from build123d import *

# Parameters (mm, degrees)
REVOLVE1_ANGLE = 180
SHELL1_START   = -239.158306138
SHELL1_DEPTH   = 42.206593174
SHELL1_START_2 = -3.058115052
SHELL1_2_DEPTH = 41.216014124
SHELL1_START_3 = -196.951712964
SHELL1_3_DEPTH = 193.893597912
SHELL1_START_4 = -221.288155922
SHELL1_4_DEPTH = 5.892364499


# Read off the part's stored shape, not the designer's step: Shell1
with BuildPart() as part:
    # Sketch1 → Revolve1 (revolve)
    with BuildSketch(Plane.XY):
        Polygon((89.874416534, -245.158306138), (12.7, -245.158306138), (12.7, -242.138884915), (26.163339875, -242.138884915), (26.163339875, -227.288155922), (13.03850974, -227.288155922), (13.03850974, -209.395791423), (26.163339875, -209.395791423), (26.163339875, -194.322320246), (13.03850974, -194.322320246), (13.03850974, -190.951712964), (73.402730944, -190.951712964), (73.402730944, -136.120329582), (15.924443856, -136.120329582), (15.924443856, -125.873058549), (73.402730944, -125.873058549), (73.402730944, -72.501855253), (16.640249143, -72.501855253), (16.640249143, -62.681553847), (73.402730944, -62.681553847), (73.402730944, -9.058115052), (18.31208302, -9.058115052), (18.31208302, -7.976977068), (29.551500324, -7.976977068), (29.551500324, 8.480345585), (18.31208302, 8.480345585), (18.31208302, 18.090461002), (29.551500324, 18.090461002), (29.551500324, 35.26854231), (18.31208302, 35.26854231), (18.31208302, 44.157899072), (89.874416534, 44.157899072), align=None)
    revolve(axis=Axis((0, 19.84375, 0), (0, 1, 0)), revolution_arc=REVOLVE1_ANGLE)

    # Shell1 outline → Shell1 (cut)
    with BuildSketch(Plane(origin=(0, 0, 0), x_dir=(1, 0, 0), z_dir=(0, 1, 0)).offset(SHELL1_START)):
        with BuildLine():
            ThreePointArc((83.874416534, 0), (0, 83.874416534), (-83.874416534, 0))
            Line((-83.874416534, 0), (-32.163339875, 0))
            ThreePointArc((-32.163339875, 0), (0, 32.163339875), (32.163339875, 0))
            Line((32.163339875, 0), (83.874416534, 0))
        make_face()
    extrude(amount=SHELL1_DEPTH, mode=Mode.SUBTRACT)

    # Shell1 2 outline → Shell1 2 (cut)
    with BuildSketch(Plane(origin=(0, 0, 0), x_dir=(1, 0, 0), z_dir=(0, 1, 0)).offset(SHELL1_START_2)):
        with BuildLine():
            ThreePointArc((83.874416534, 0), (0, 83.874416534), (-83.874416534, 0))
            Line((-83.874416534, 0), (-35.551500324, 0))
            ThreePointArc((-35.551500324, 0), (0, 35.551500324), (35.551500324, 0))
            Line((35.551500324, 0), (83.874416534, 0))
        make_face()
    extrude(amount=SHELL1_2_DEPTH, mode=Mode.SUBTRACT)

    # Shell1 3 outline → Shell1 3 (cut)
    with BuildSketch(Plane(origin=(0, 0, 0), x_dir=(1, 0, 0), z_dir=(0, 1, 0)).offset(SHELL1_START_3)):
        with BuildLine():
            ThreePointArc((83.874416534, 0), (0, 83.874416534), (-83.874416534, 0))
            Line((-83.874416534, 0), (-79.402730944, 0))
            ThreePointArc((-79.402730944, 0), (0, 79.402730944), (79.402730944, 0))
            Line((79.402730944, 0), (83.874416534, 0))
        make_face()
    extrude(amount=SHELL1_3_DEPTH, mode=Mode.SUBTRACT)

    # Shell1 4 outline → Shell1 4 (cut)
    with BuildSketch(Plane(origin=(0, 0, 0), x_dir=(1, 0, 0), z_dir=(0, 1, 0)).offset(SHELL1_START_4)):
        with BuildLine():
            ThreePointArc((32.163339875, 0), (0, 32.163339875), (-32.163339875, 0))
            Line((-32.163339875, 0), (-19.03850974, 0))
            ThreePointArc((-19.03850974, 0), (0, 19.03850974), (19.03850974, 0))
            Line((19.03850974, 0), (32.163339875, 0))
        make_face()
    extrude(amount=SHELL1_4_DEPTH, mode=Mode.SUBTRACT)


solid = part.part
Geometry: final body of the model. Coordinates: model frame, mm. A direction names the side the tool comes from. Give positions to 0.01 mm unless a question says otherwise; leave off trailing zeros. Write each loop counter-clockwise with the first axis right and the second up, starting at its lowest first coordinate (ties: lowest second). Pieces come first, ordered by that corner, then holes. Notation, with made-up numbers: (61.5, 22) -> (82.5, 22) arc R20 cw to (82.5, 60) -> close; hole circle Ø6 at (87, 65). An arc over 180 degrees is marked (long way). Answer as a JSON object with one key per item and string values.
1. Cut plane A-A on z = -60.5. Output: boundary loops of the cut face in (x, y).
Ans:
{"outline": "(-66.46, -245.16) -> (66.46, -245.16) -> (66.46, 44.16) -> (-66.46, 44.16) -> close; (-51.43, -196.95) -> (51.43, -196.95) -> (51.43, -3.06) -> (-51.43, -3.06) -> close; hole (-58.09, -239.16) -> (58.09, -239.16) -> (58.09, 38.16) -> (-58.09, 38.16) -> close; hole (-41.57, -190.95) -> (41.57, -190.95) -> (41.57, -136.12) -> (-41.57, -136.12) -> close; hole (-41.57, -125.87) -> (41.57, -125.87) -> (41.57, -72.5) -> (-41.57, -72.5) -> close; hole (-41.57, -62.68) -> (41.57, -62.68) -> (41.57, -9.06) -> (-41.57, -9.06) -> close"}
2. Contact query for flat-ended pins moving along their axis: pin 1 (8 mm diameter, centred on x = 9.5, y = -44, fed in from +Z); pin 2 (2 mm diameter, centred on x = -51, y = -94, fed in from -Z); pin 3 (6 mm diameter, centred on y = -41, z = -62.5, fed in from +X). Output: stop coordinate, or through.
Ans:
{"pin 1": "stops at z = -72.15", "pin 2": "stops at z = -74.68", "pin 3": "stops at x = 67.36"}
3. Mould query, pull axis Y, two halves, no side actions, for faces 4 (the flat face through (-1, -245.158, -36)), 5 (the cylindrical face through (0.403, -8.51, -18.308)), 6 (the flat face through (0.4, -209.396, -13.3)). Classes: pulls with the +Y half, pulls with the -Y half, needs draft (parallel to the pull), parting line crosses it, or undercut.
Ans:
{"face 4": "pulls with the -Y half", "face 5": "needs draft", "face 6": "undercut"}
4. Cut plane B-B on y = 26.5. Output: boundary loops of the cut face in (x, z), and give its area (3 significant figures).
Ans:
{"outline": "(-89.87, 0) arc R89.87 ccw to (89.87, 0) -> (83.87, 0) arc R83.87 cw to (-83.87, 0) -> close; (-35.55, 0) arc R35.55 ccw to (35.55, 0) -> (29.55, 0) arc R29.55 cw to (-29.55, 0) -> close", "area": "2,250 mm^2"}
5. Access query for faces 1 (the cylindrical face through (0.287, -192.613, -13.035)), 2 (the flat face through (0, 18.09, -22)), 3 (the cylindrical face through (-0.707, -230.348, -32.156)). Directions: +Z, -Z, +X, -X, +Y, -Y. A direction counts if a zero-diameter tool reaches every point of the face in a straight line with its end or side. Return the directions, or none.
Ans:
{"face 1": "+Z, +Y", "face 2": "+Z", "face 3": "none"}
6. Ray query, probe 1 along Y at (x, z) = (-16.5, -5); probe 2 along Y at (x, z) = (-70, -9); probe 3 along Z at (x, y) = (1.5, -125). Return the intervals inside material, ascending. Write a range as from..to.
Ans:
{"probe 1": "y = -245.16..-242.14, -227.29..-209.4, -194.32..-190.95, -136.12..-125.87, -72.5..-62.68", "probe 2": "y = -245.16..-239.16, -196.95..-190.95, -136.12..-125.87, -72.5..-62.68, -9.06..-3.06, 38.16..44.16", "probe 3": "z = -89.86..-83.86, -79.39..-73.39"}
7. Cut plane D-D on y = -102.5. Output: boundary loops of the cut face in (x, z).
Ans:
{"outline": "(-89.87, 0) arc R89.87 ccw to (89.87, 0) -> (83.87, 0) arc R83.87 cw to (-83.87, 0) -> close; (-79.4, 0) arc R79.4 ccw to (79.4, 0) -> (73.4, 0) arc R73.4 cw to (-73.4, 0) -> close"}
8. Cut plane C-C on x = -58.5. Output: boundary loops of the cut face in (y, z), and give its area (3 significant figures).
Ans:
{"outline": "(-245.16, -68.23) -> (44.16, -68.23) -> (44.16, 0) -> (38.16, 0) -> (38.16, -60.11) -> (-239.16, -60.11) -> (-239.16, 0) -> (-245.16, 0) -> close; (-196.95, -53.69) -> (-3.06, -53.69) -> (-3.06, 0) -> (-9.06, 0) -> (-9.06, -44.34) -> (-62.68, -44.34) -> (-62.68, 0) -> (-72.5, 0) -> (-72.5, -44.34) -> (-125.87, -44.34) -> (-125.87, 0) -> (-136.12, 0) -> (-136.12, -44.34) -> (-190.95, -44.34) -> (-190.95, 0) -> (-196.95, 0) -> close", "area": "6,310 mm^2"}
